```python
from build123d import *

# Parameters (mm, degrees)
SKETCH1_R           = 12.5
BOSS_EXTRUDE1_DEPTH = 148.5
SKETCH2_OUTSIDE_W   = 57.53
SKETCH2_OUTSIDE_H   = 57.53
SKETCH2_OUTSIDE_R   = 8
CUT_EXTRUDE1_DEPTH  = 121.5
SKETCH3_OUTSIDE_W   = 57.53
SKETCH3_OUTSIDE_H   = 57.53
SKETCH3_OUTSIDE_R   = 1.875
CUT_EXTRUDE2_DEPTH  = 8
FILLET1_R           = 4
FILLET2_R           = 7
SKETCH6_OUTSIDE_W   = 57.53
SKETCH6_OUTSIDE_H   = 57.53
SKETCH6_OUTSIDE_R   = 11.75
CUT_EXTRUDE3_DEPTH  = 2.2
FILLET3_R           = 0.25


with BuildPart() as part:
    # Sketch1 → Boss-Extrude1 (new body)
    with BuildSketch(Plane(origin=(0, 0, 0), x_dir=(1, 0, 0), z_dir=(0, 1, 0))):
        with Locations(Location((0, 0, 0), (0, 0, 270))):
            Circle(SKETCH1_R)
    extrude(amount=BOSS_EXTRUDE1_DEPTH)

    # Sketch2 outside → Cut-Extrude1 (cut)
    with BuildSketch(Plane.XZ):
        Rectangle(SKETCH2_OUTSIDE_W, SKETCH2_OUTSIDE_H)
        with Locations(Location((0, 0, 0), (0, 0, 270))):
            Circle(SKETCH2_OUTSIDE_R, mode=Mode.SUBTRACT)
    extrude(amount=-CUT_EXTRUDE1_DEPTH, mode=Mode.SUBTRACT)

    # Sketch3 outside → Cut-Extrude2 (cut)
    with BuildSketch(Plane(origin=(0, 148.5, 0), x_dir=(1, 0, 0), z_dir=(0, 1, 0))):
        Rectangle(SKETCH3_OUTSIDE_W, SKETCH3_OUTSIDE_H)
        with Locations(Location((0, 0, 0), (0, 0, 270))):
            Circle(SKETCH3_OUTSIDE_R, mode=Mode.SUBTRACT)
    extrude(amount=-CUT_EXTRUDE2_DEPTH, mode=Mode.SUBTRACT)

    # Fillet1
    fillet1_edges = [part.edges().sort_by_distance(p)[0] for p in [
        (0, 121.5, -12.5),
    ]]
    fillet(fillet1_edges, radius=FILLET1_R)

    # Fillet2
    fillet2_edges = [part.edges().sort_by_distance(p)[0] for p in [
        (0, 0, 8),
    ]]
    fillet(fillet2_edges, radius=FILLET2_R)

    # Sketch6 outside → Cut-Extrude3 (cut)
    with BuildSketch(Plane(origin=(0, 140.5, 0), x_dir=(1, 0, 0), z_dir=(0, 1, 0))):
        Rectangle(SKETCH6_OUTSIDE_W, SKETCH6_OUTSIDE_H)
        with Locations(Location((0, 0, 0), (0, 0, 270))):
            Circle(SKETCH6_OUTSIDE_R, mode=Mode.SUBTRACT)
    extrude(amount=-CUT_EXTRUDE3_DEPTH, mode=Mode.SUBTRACT)

    # Fillet3
    fillet3_edges = [part.edges().sort_by_distance(p)[0] for p in [
        (0, 138.3, -11.75),
        (0, 138.3, -12.5),
        (0, 140.5, -11.75),
    ]]
    fillet(fillet3_edges, radius=FILLET3_R)


solid = part.part
```
Check sheet for the modelled part. Datum: model origin and axes. Units: mm. A direction names the side the tool comes from. Round coordinates to 2 decimals unless told otherwise and drop trailing zeros. Order: outer loops, then holes, each group sorted by start corner. A loop starts at its lowest first (then second) coordinate and runs counter-clockwise, first axis right, second up. Notation, with made-up numbers: M 22,-27 L 59,-27 A31 cw 59,-2 Z; hole C -11.5,-3.5 d7. An arc over 180 degrees is marked long. Answer in a Markdown table with one row per item.
(1) Section check A-A on y = 22. Record the boundary of the cut face in (x, z).
Findings:
| item | result |
|---|---|
| outline | C 0,0 d16 |
(2) Section check B-B on y = 130. Record the boundary of the cut face in (x, z), plus the area to 3 significant figures.
Findings:
| item | result |
|---|---|
| outline | C 0,0 d25 |
| area | 491 mm^2 |
(3) Set-up check for faces 1 (the cylindrical face through (0.082, 144.556, -1.873)), 2 (the cylindrical face through (-7.81, 63.45, 1.73)), 3 (the cylindrical face through (3.755, 131.687, 11.923)): record each of +Z, -Z, +X, -X, +Y, -Y from which the full face is reachable in a straight line by a thin tool's end or side.
Findings:
| item | result |
|---|---|
| face 1 | +Y |
| face 2 | -Y |
| face 3 | +Y, -Y |
(4) Gauge pin test, flat ends, axial feed: pin 1 (12 mm diameter, centred on x = -8.5, z = -8.5, fed in from -Y); pin 2 (6 mm diameter, centred on x = -8.5, y = 103, fed in from -Z); pin 3 (10 mm diameter, centred on x = 4.5, z = -1, fed in from +Y); pin 4 (12 mm diameter, centred on x = 2.5, y = 83, fed in from +Z). Record the tip position at first contact, or that the pin passes through.
Findings:
| item | result |
|---|---|
| pin 1 | stops at y = 2.12 |
| pin 2 | stops at z = -5.81 |
| pin 3 | stops at y = 148.5 |
| pin 4 | stops at z = 8 |
(5) Material ranges on line 1 along Z through (x, y) = (-0.25, 133); line 2 along Y through (x, z) = (6, 6.5); line 3 along X through (y, z) = (39, 0), recorded low to high. Write a range as from..to.
Findings:
| item | result |
|---|---|
| line 1 | z = -12.5..12.5 |
| line 2 | y = 121.51..140.5 |
| line 3 | x = -8..8 |
